```python
from build123d import *

# Parameters (mm, degrees)
SKETCH1_R           = 24.75
BOSS_EXTRUDE1_DEPTH = 42.5
SKETCH2_R           = 4
BOSS_EXTRUDE2_DEPTH = 2.5
SKETCH6_R           = 2
CUT_EXTRUDE3_DEPTH  = 5
CIRPATTERN1_COUNT   = 4
SKETCH5_R           = 2
CUT_EXTRUDE2_DEPTH  = 10
CIRPATTERN2_COUNT   = 4
SKETCH7_R           = 10.5
BOSS_EXTRUDE3_DEPTH = 5


with BuildPart() as part:
    # Sketch1 → Boss-Extrude1 (new body, symmetric)
    with BuildSketch(Plane.XY):
        Circle(SKETCH1_R)
    extrude(amount=BOSS_EXTRUDE1_DEPTH, both=True)

    # Sketch2 → Boss-Extrude2 (add)
    with BuildSketch(Plane.XY.offset(42.5)):
        Circle(SKETCH2_R)
    extrude(amount=BOSS_EXTRUDE2_DEPTH)

    # Sketch6 → Cut-Extrude3 (cut)
    with BuildSketch(Plane.XY.offset(42.5)):
        with Locations((0, 17.5)):
            Circle(SKETCH6_R)
    cut_extrude3 = extrude(amount=-CUT_EXTRUDE3_DEPTH, mode=Mode.SUBTRACT)

    # CirPattern1: Cut-Extrude3 ×4 about axis
    cirpattern1_axis = Axis((0, 0, 0), (0, 0, 1))
    for i in range(1, CIRPATTERN1_COUNT):
        add(cut_extrude3.rotate(cirpattern1_axis, i * 360 / CIRPATTERN1_COUNT), mode=Mode.SUBTRACT)

    # Sketch5 → Cut-Extrude2 (cut)
    with BuildSketch(Plane(origin=(0, 0, -42.5), x_dir=(-1, 0, 0), z_dir=(0, 0, -1))):
        with Locations((-17.5, 0)):
            Circle(SKETCH5_R)
    cut_extrude2 = extrude(amount=-CUT_EXTRUDE2_DEPTH, mode=Mode.SUBTRACT)

    # CirPattern2: Cut-Extrude2 ×4 about axis
    cirpattern2_axis = Axis((0, 0, 0), (0, 0, 1))
    for i in range(1, CIRPATTERN2_COUNT):
        add(cut_extrude2.rotate(cirpattern2_axis, i * 360 / CIRPATTERN2_COUNT), mode=Mode.SUBTRACT)

    # Sketch7 → Boss-Extrude3 (add)
    with BuildSketch(Plane(origin=(0, 0, -42.5), x_dir=(-1, 0, 0), z_dir=(0, 0, -1))):
        Circle(SKETCH7_R)
    extrude(amount=BOSS_EXTRUDE3_DEPTH)


solid = part.part
```
The listing builds one solid part. Answer for the finished solid, in the listing's coordinates (mm). A direction names the side the tool comes from. Round coordinates to 2 decimals unless told otherwise and drop trailing zeros. Order: outer loops, then holes, each group sorted by start corner. A loop starts at its lowest first (then second) coordinate and runs counter-clockwise, first axis right, second up. Notation, with made-up numbers: (77.25, -40) -> (95.25, -40) arc R21 cw to (95.25, -2) -> close; hole circle Ø2 at (56.25, 9.5). An arc over 180 degrees is marked (long way). Answer as CSV lines item,"result". Start each with the question number.
(1) Flat-ended cylindrical pins translate along their axes: pin 1 Ø3 at (x, y) = (17.5, 0) entering from -Z; pin 2 Ø3 at (x, y) = (1, 18.5) entering from -Z; pin 3 Ø3 at (x, y) = (0, 17.5) entering from +Z; pin 4 Ø25 at (x, y) = (-11, 6) entering from -Z. Find the tip coordinate at first contact, or state that the pin passes through.
(2) The part is cut by section D-D (z = -25). Determine the outline of the cut face in (x, y), then the cut area to 3 significant figures.
(3) A tool of negligible diameter and unlimited length cuts with its end or side. For faces 1 (the face through (-18, 0, -32.5)), 2 (the face through (19.483, 0.26, 40.035)), 3 (the face through (-3.22, 24.54, 0.59)), from which of +Z, -Z, +X, -X, +Y, -Y can it reach the whole face along a straight path? Write none if from no direction.
(4) Find the intervals of material crossed by probe 1 along Y at (x, z) = (0, 39.6); probe 2 along Z at (x, y) = (18.5, 6); probe 3 along X at (y, z) = (-17.5, 39.95), in increasing order. Write a range as from..to.
(5) For a pull along Y with two mould halves and no side action, classify faces 4 (the face through (0, 0, 45)), 5 (the face through (18, 0, 37.5)), 6 (the face through (-0.867, -3.905, 43.732)) as +Y half, -Y half, draft (parallel to the pull), parting line (faces both ways), or undercut.
(6) The part is cut by section B-B (x = 0). Determine the outline of the cut face in (y, z), then the cut area to 3 significant figures.
(7) The part is cut by section A-A (z = 39.5). Determine the outline of the cut face in (x, y), then the cut area to 3 significant figures.
Evaluation:
1,pin 1,"z = -32.5"
1,pin 2,"z = -42.5"
1,pin 3,"z = 37.5"
1,pin 4,"z = -47.5"
2,outline,"circle Ø49.5 at (0, 0)"
2,area,"1,920 mm²"
3,face 1,"-Z"
3,face 2,"+Z"
3,face 3,"+Z, -Z"
4,probe 1,"-24.75..-19.5, -15.5..15.5, 19.5..24.75"
4,probe 2,"-42.5..42.5"
4,probe 3,"-17.5..-2, 2..17.5"
5,face 4,"draft"
5,face 5,"undercut"
5,face 6,"parting line"
6,outline,"(-24.75, -42.5) -> (-19.5, -42.5) -> (-19.5, -32.5) -> (-15.5, -32.5) -> (-15.5, -42.5) -> (-10.5, -42.5) -> (-10.5, -47.5) -> (10.5, -47.5) -> (10.5, -42.5) -> (15.5, -42.5) -> (15.5, -32.5) -> (19.5, -32.5) -> (19.5, -42.5) -> (24.75, -42.5) -> (24.75, 42.5) -> (19.5, 42.5) -> (19.5, 37.5) -> (15.5, 37.5) -> (15.5, 42.5) -> (4, 42.5) -> (4, 45) -> (-4, 45) -> (-4, 42.5) -> (-15.5, 42.5) -> (-15.5, 37.5) -> (-19.5, 37.5) -> (-19.5, 42.5) -> (-24.75, 42.5) -> close"
6,area,"4,210 mm²"
7,outline,"circle Ø49.5 at (0, 0); hole circle Ø4 at (-17.5, 0); hole circle Ø4 at (0, -17.5); hole circle Ø4 at (0, 17.5); hole circle Ø4 at (17.5, 0)"
7,area,"1,870 mm²"
